Read the model definition and answer for the solid it produces. Units are mm, in the model's axes. Face numbers are marked on the shaded views. A direction names the side the tool comes from. Coordinates: 2 decimals unless noted, no trailing zeros. Write each loop counter-clockwise with the first axis right and the second up, starting at its lowest first coordinate (ties: lowest second). Pieces come first, ordered by that corner, then holes. Notation, with made-up numbers: (71.5, 79) -> (111.5, 79) arc R28 cw to (111.5, 117) -> close; hole circle Ø8 at (-5, 42.25). An arc over 180 degrees is marked (long way). Answer as a JSON object with one key per item and string values. Group by question number.
(1) Which of the six approach directions +Z, -Z, +X, -X, +Y, -Y give full straight-line access (tool end or side, diameter ignored) to the marked faces 4 and 5?
(2) A flat-ended cylindrical pin translates along its axis: P1, Ø7.5, axis at x = 2, z = -1.5, coming from the +Y side. Find the tip coordinate at first contact, or state that the pin passes through.
(3) Find section D-D (z = -3.5). Give the vertices of the cut face in (x, y).
(4) Find section C-C (x = -5.5). Give the vertices of the cut face in (y, z), then the cut area to 3 significant figures.
(5) Find section A-A (y = 5.75). Give the vertices of the cut face in (x, z), then the cut area to 3 significant figures.
(6) Find section B-B (z = 5). Give the vertices of the cut face in (x, y).
(7) Straight lines are drawn through the part: L1, parallel to X at y = 2.1, z = 0; L2, parallel to X at y = 4, z = 0. For each, find the intervals that lie inside material, in ascending order.
(8) For a pull along X with two mould halves and no side action, classify the marked faces 1, 2 and 3 as +X half, -X half, draft (parallel to the pull), parting line (faces both ways), or undercut.
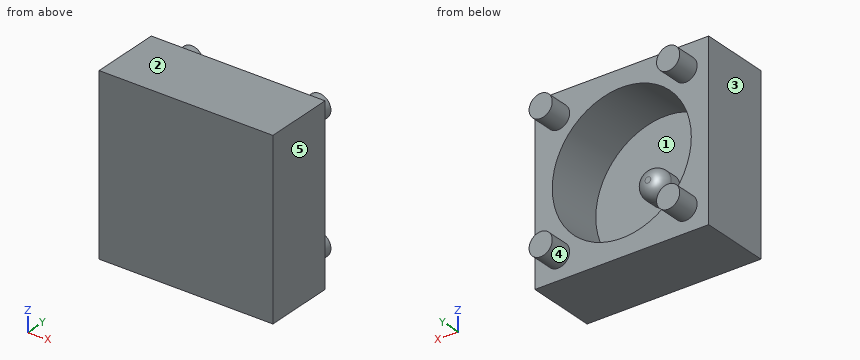
from build123d import *

# Parameters (mm, degrees)
SKETCH1_W           = 15
SKETCH1_H           = 15
BOSS_EXTRUDE1_DEPTH = 6
SKETCH2_R           = 6
CUT_EXTRUDE1_DEPTH  = 5
SKETCH3_R           = 1.25
BOSS_EXTRUDE2_DEPTH = 2
FILLET1_R           = 1
SKETCH4_R           = 1
BOSS_EXTRUDE3_DEPTH = 2


with BuildPart() as part:
    # Sketch1 → Boss-Extrude1 (new body)
    with BuildSketch(Plane(origin=(0, 0, 0), x_dir=(1, 0, 0), z_dir=(0, 1, 0))):
        Rectangle(SKETCH1_W, SKETCH1_H)
    extrude(amount=BOSS_EXTRUDE1_DEPTH)

    # Sketch2 → Cut-Extrude1 (cut)
    with BuildSketch(Plane(origin=(0, 6, 0), x_dir=(1, 0, 0), z_dir=(0, 1, 0))):
        Circle(SKETCH2_R)
    extrude(amount=-CUT_EXTRUDE1_DEPTH, mode=Mode.SUBTRACT)

    # Sketch3 → Boss-Extrude2 (add)
    with BuildSketch(Plane(origin=(0, 1, 0), x_dir=(1, 0, 0), z_dir=(0, 1, 0))):
        Circle(SKETCH3_R)
    extrude(amount=BOSS_EXTRUDE2_DEPTH)

    # Fillet1
    fillet1_edges = [part.edges().sort_by_distance(p)[0] for p in [
        (-1.25, 3, 0),
    ]]
    fillet(fillet1_edges, radius=FILLET1_R)

    # Sketch4 → Boss-Extrude3 (add)
    with BuildSketch(Plane(origin=(0, 6, 0), x_dir=(1, 0, 0), z_dir=(0, 1, 0))):
        with Locations((-5.5, 5.5)):
            Circle(SKETCH4_R)
        with Locations((5.5, 5.5)):
            Circle(SKETCH4_R)
        with Locations((-5.5, -5.5)):
            Circle(SKETCH4_R)
        with Locations((5.5, -5.5)):
            Circle(SKETCH4_R)
    extrude(amount=BOSS_EXTRUDE3_DEPTH)


solid = part.part
Results below:
{
 "1": {"face 4": "+Y", "face 5": "+Z, -Z, +X, +Y, -Y"},
 "2": {"P1": "stops at y = 6"},
 "3": {"outline": "(-7.5, 0) -> (7.5, 0) -> (7.5, 6) -> (4.87, 6) -> (4.87, 1) -> (-4.87, 1) -> (-4.87, 6) -> (-7.5, 6) -> close"},
 "4": {"outline": "(0, -7.5) -> (6, -7.5) -> (6, -6.5) -> (8, -6.5) -> (8, -4.5) -> (6, -4.5) -> (6, -2.4) -> (1, -2.4) -> (1, 2.4) -> (6, 2.4) -> (6, 4.5) -> (8, 4.5) -> (8, 6.5) -> (6, 6.5) -> (6, 7.5) -> (0, 7.5) -> close", "area": "74.0 mm2"},
 "5": {"outline": "(-7.5, -7.5) -> (7.5, -7.5) -> (7.5, 7.5) -> (-7.5, 7.5) -> close; hole circle Ø12 at (0, 0)", "area": "112 mm2"},
 "6": {"outline": "(-7.5, 0) -> (7.5, 0) -> (7.5, 6) -> (6.37, 6) -> (6.37, 8) -> (4.63, 8) -> (4.63, 6) -> (3.32, 6) -> (3.32, 1) -> (-3.32, 1) -> (-3.32, 6) -> (-4.63, 6) -> (-4.63, 8) -> (-6.37, 8) -> (-6.37, 6) -> (-7.5, 6) -> close"},
 "7": {"L1": "x = -7.5 to -6, -1.24 to 1.24, 6 to 7.5", "L2": "x = -7.5 to -6, 6 to 7.5"},
 "8": {"face 1": "undercut", "face 2": "draft", "face 3": "-X half"}
}
